from build123d import *

# Parameters (mm, degrees)
F0_R     = 3.937
F1_DEPTH = 1.016
F2_R     = 2.413
F3_DEPTH = 1.778
F4_R     = 3.175
F4_R_2   = 2.413
F5_DEPTH = 2.3622


with BuildPart() as f1:
    # F0 (on Top) → F1 (new body)
    with BuildSketch(Plane.XY):
        Circle(F0_R)
    extrude(amount=F1_DEPTH)

    # F2 (on face) → F3 (join)
    with BuildSketch(Plane.XY.offset(1.016)):
        Circle(F2_R)
    extrude(amount=F3_DEPTH)

    # F4 (on face) → F5 (join)
    with BuildSketch(Plane(origin=(0, 0, 0), x_dir=(1, 0, 0), z_dir=(0, 0, -1))):
        Circle(F4_R)
        Circle(F4_R_2, mode=Mode.SUBTRACT)
    extrude(amount=F5_DEPTH)


solid = f1.part
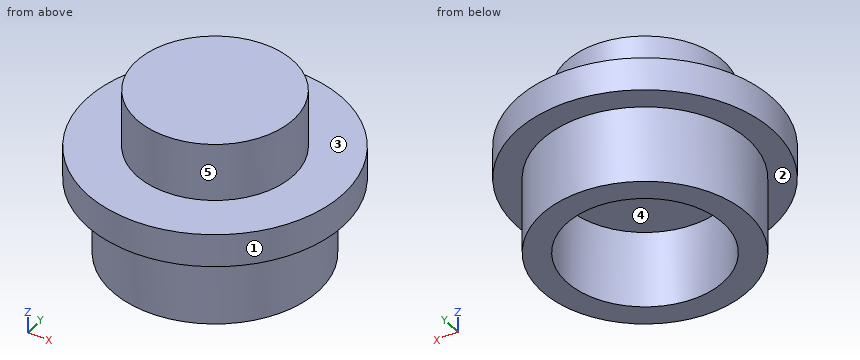
CAD build for the part. Positions are in the model's coordinates, mm. Face numbers are marked on the shaded views. A direction names the side the tool comes from. Give positions to 0.01 mm unless a question says otherwise; leave off trailing zeros. Write each loop counter-clockwise with the first axis right and the second up, starting at its lowest first coordinate (ties: lowest second). Pieces come first, ordered by that corner, then holes. Notation, with made-up numbers: M 66,63.5 L 120,63.5 A14 ccw 120,90.5 Z; hole C -26.75,-35.75 d4. An arc over 180 degrees is marked long. Put each result on its own line as item: value. Start each with the question number.
(1) Band-saw the part on A-A, the plane x = 0. Write the cut outline in (y, z) (3 decimals), and give its area (3 significant figures).
(2) Band-saw the part on B-B, the plane z = -1.4. Write the cut outline in (x, y) (3 decimals), and give its area (3 significant figures).
(3) Mould opens along X. For the marked faces 3, 4 and 5 say: +X half, -X half, draft (parallel to the pull), parting line (faces both ways), or undercut.
(4) Flat gauge pins, fed straight in: pin 1 Ø1 at (y, z) = (0.5, 0.5) entering from +X; pin 2 Ø1.5 at (x, z) = (3, 1.5) entering from -Y; pin 3 Ø1.5 at (x, z) = (-1, 1.5) entering from -Y; pin 4 Ø3 at (y, z) = (-2, 0) entering from -X. Where does each tip first touch, or does it go through?
(5) Which spindle directions (+Z, -Z, +X, -X, +Y, -Y) get a long thin tool onto all of the face, cutting with end or side? Do the marked faces 1 and 2. Say none if no direction does.
(6) Probe L1, parallel to Y at x = 0, z = -1.45 (3 decimals); L2, parallel to Z at x = 2, y = 0.5. List the from-to ranges inside material, lowest first.
Response values:
1. outline: M -3.937,0 L -3.175,0 L -3.175,-2.362 L -2.413,-2.362 L -2.413,0 L 2.413,0 L 2.413,-2.362 L 3.175,-2.362 L 3.175,0 L 3.937,0 L 3.937,1.016 L 2.413,1.016 L 2.413,2.794 L -2.413,2.794 L -2.413,1.016 L -3.937,1.016 Z
1. area: 20.2 mm2
2. outline: C 0,0 d6.35; hole C 0,0 d4.826
2. area: 13.4 mm2
3. face 3: draft
3. face 4: undercut
3. face 5: parting line
4. pin 1: stops at x = 3.94
4. pin 2: stops at y = -3.1
4. pin 3: stops at y = -3.91
4. pin 4: stops at x = -3.91
5. face 1: +Z, -Z
5. face 2: -Z
6. L1: y = -3.175 to -2.413, 2.413 to 3.175
6. L2: z = 0 to 2.79
